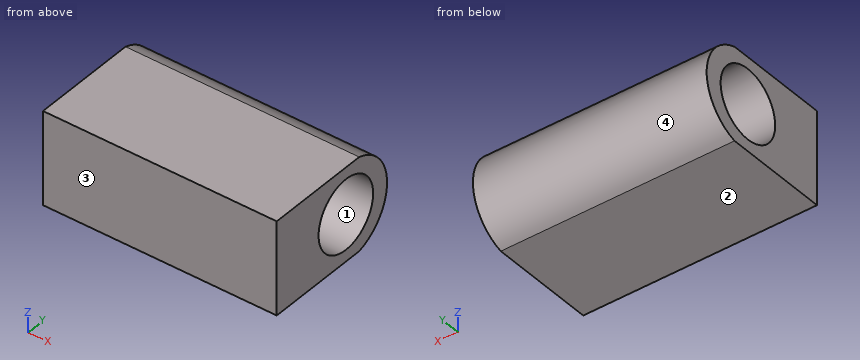
```python
from build123d import *

# Parameters (mm, degrees)
SKETCH1_W               = 50
SKETCH1_H               = 20
BOSS_EXTRUDE1_DEPTH     = 44
SKETCH3_R               = 7.5
CUT_EXTRUDE3_DEPTH      = 26
CUT_EXTRUDE3_DEPTH_BACK = 26
CUT_EXTRUDE4_DEPTH      = 26
CUT_EXTRUDE4_DEPTH_BACK = 26


with BuildPart() as part:
    # Sketch1 → Boss-Extrude1 (new body)
    with BuildSketch(Plane(origin=(0, 0, 0), x_dir=(1, 0, 0), z_dir=(0, 1, 0))):
        Rectangle(SKETCH1_W, SKETCH1_H)
    extrude(amount=BOSS_EXTRUDE1_DEPTH)

    # Sketch3 → Cut-Extrude3 (cut, two sides)
    with BuildSketch(Plane(origin=(0, 0, 0), x_dir=(0, 0, -1), z_dir=(1, 0, 0))) as cut_extrude3_sk:
        with Locations((0, 19)):
            Circle(SKETCH3_R)
    extrude(amount=CUT_EXTRUDE3_DEPTH, mode=Mode.SUBTRACT)
    extrude(cut_extrude3_sk.sketch, amount=-CUT_EXTRUDE3_DEPTH_BACK, mode=Mode.SUBTRACT)

    # Sketch4 → Cut-Extrude4 (cut, two sides)
    with BuildSketch(Plane(origin=(0, 0, 0), x_dir=(0, 0, -1), z_dir=(1, 0, 0))) as cut_extrude4_sk:
        with BuildLine():
            Line((-10, 22.677289201), (-10, 44))
            Line((-10, 44), (10, 44))
            Line((10, 44), (10, 22.677289201))
            ThreePointArc((10, 22.677289201), (0, 30.338307173), (-10, 22.677289201))
        make_face()
    extrude(amount=CUT_EXTRUDE4_DEPTH, mode=Mode.SUBTRACT)
    extrude(cut_extrude4_sk.sketch, amount=-CUT_EXTRUDE4_DEPTH_BACK, mode=Mode.SUBTRACT)


solid = part.part
```
CAD build for the part. Positions are in the model's coordinates, mm. Face numbers are marked on the shaded views. Round coordinates to 2 decimals unless told otherwise and drop trailing zeros. Order: outer loops, then holes, each group sorted by start corner. A loop starts at its lowest first (then second) coordinate and runs counter-clockwise, first axis right, second up. Notation, with made-up numbers: (12.25, 43.5) - (62.25, 43.5) arc R19 cw to (62.25, 67.5) - close; hole circle Ø2 at (-1.5, -35). An arc over 180 degrees is marked (long way). Use CSV: the item, a comma, the result in double quotes. Start each with the question number.
1) Wall check: L1, parallel to Y at x = -9.5, z = 0; L2, parallel to Z at x = 12, y = 19; L3, parallel to Z at x = -12, y = 25. Give the ranges that are in metal, low to high. Write a range as [from, to].
2) Saw through at D-D (y = 28). List the corners of the cut face in (x, z).
3) Pin check, flat tip, straight feed: pin 1 Ø1.5 at (y, z) = (12.5, -1.5) entering from +X. Stop position of the tip, or through.
4) Two-plate mould, pull along Y, no slides. Class the marked faces 1, 2, 3 and 4: pulls with the +Y half, pulls with the -Y half, needs draft (parallel to the pull), parting line crosses it, or undercut.
5) Saw through at C-C (x = -15.5). List the corners of the cut face in (y, z).
6) Saw through at B-B (z = 4). List the corners of the cut face in (x, y), and give its area (3 significant figures).
7) Saw through at A-A (y = 19). List the corners of the cut face in (x, z), and give its area (3 significant figures).
Values follow:
1,L1,"y = [0, 11.5], [26.5, 30.34]"
1,L2,"z = [-10, -7.5], [7.5, 10]"
1,L3,"z = [-9.06, -4.5], [4.5, 9.06]"
2,outline,"(-25, -6.56) - (25, -6.56) - (25, 6.56) - (-25, 6.56) - close"
3,pin 1,"passes through"
4,face 1,"undercut"
4,face 2,"needs draft"
4,face 3,"pulls with the -Y half"
4,face 4,"pulls with the +Y half"
5,outline,"(0, -10) - (22.68, -10) arc R10.36 ccw to (22.68, 10) - (0, 10) - close; hole circle Ø15 at (19, 0)"
6,outline,"(-25, 0) - (25, 0) - (25, 12.66) - (-25, 12.66) - close; (-25, 25.34) - (25, 25.34) - (25, 29.53) - (-25, 29.53) - close"
6,area,"842 mm2"
7,outline,"(-25, -10) - (25, -10) - (25, -7.5) - (-25, -7.5) - close; (-25, 7.5) - (25, 7.5) - (25, 10) - (-25, 10) - close"
7,area,"250 mm2"
